Read the model definition and answer for the solid it produces. Units are mm, in the model's axes. Round coordinates to 2 decimals unless told otherwise and drop trailing zeros. Write each loop counter-clockwise with the first axis right and the second up, starting at its lowest first coordinate (ties: lowest second). Pieces come first, ordered by that corner, then holes. Notation, with made-up numbers: (-25.75, 89) - (-21.75, 89) arc R18 cw to (-21.75, 118) - close; hole circle Ø3 at (88, 43.5). An arc over 180 degrees is marked (long way). Answer as CSV lines item,"result". Start each with the question number.
1) Find section B-B on z = 57. Determine the outline of the cut face in (x, y), then the cut area to 3 significant figures.
2) Consider line 1 along Y through (x, z) = (1.8, 78.25); line 2 along Z through (x, y) = (3.55, 5); line 3 along Y through (x, z) = (7, 35.5). Determine where each line is inside the solid, lowest interval first.
3) Each of these flat-tipped pins is pushed along its axis until it touches: pin 1 (1.5 mm diameter, centred on y = 5, z = 8.25, fed in from -X); pin 2 (2 mm diameter, centred on x = 4.25, y = 40.1, fed in from -Z); pin 3 (0.5 mm diameter, centred on y = 34, z = 40.5, fed in from +X). Where does it stop, or does it pass through?
4) Find section A-A on x = 7.25. Determine the outline of the cut face in (y, z).
from build123d import *

# Parameters (mm, degrees)
BOSS_EXTRUDE1_DEPTH            = 86.5
M3X0_5_TAPPED_HOLE2_AT_2_COUNT = 2
M3X0_5_TAPPED_HOLE2_AT_2_PITCH = 23.4
M3X0_5_TAPPED_HOLE1_AT_2_COUNT = 2
M3X0_5_TAPPED_HOLE1_AT_2_PITCH = 46.8


with BuildPart() as part:
    # Sketch1 → Boss-Extrude1 (new body)
    with BuildSketch(Plane.XY):
        Polygon((0, 0), (0, 56.8), (8.5, 56.8), (8.5, 46.8), (2.5, 46.8), (2.5, 45.1), (8.5, 45.1), (8.5, 35.1), (2.5, 35.1), (2.5, 33.4), (8.5, 33.4), (8.5, 23.4), (2.5, 23.4), (2.5, 21.7), (8.5, 21.7), (8.5, 11.7), (2.5, 11.7), (2.5, 10), (8.5, 10), (8.5, 0), align=None)
    extrude(amount=BOSS_EXTRUDE1_DEPTH)

    # Sketch4 → M3x0.5 Tapped Hole2 (revolve, cut)
    with BuildSketch(Plane(origin=(4.25, 40.1, 86.5), x_dir=(0, -1, 0), z_dir=(1, 0, 0))):
        Polygon((0, 0), (0, 5.751075774), (1.25, 5), (1.25, 0), align=None)
    m3x0_5_tapped_hole2 = revolve(axis=Axis((4.25, 40.1, 92.85), (0, 0, -1)), mode=Mode.SUBTRACT)

    # M3x0.5 Tapped Hole2 at 2: M3x0.5 Tapped Hole2 ×2
    with Locations(*[(0, -i * M3X0_5_TAPPED_HOLE2_AT_2_PITCH, 0) for i in range(1, M3X0_5_TAPPED_HOLE2_AT_2_COUNT)]):
        add(m3x0_5_tapped_hole2, mode=Mode.SUBTRACT)

    # Mirror1: M3x0.5 Tapped Hole2 across plane
    add(m3x0_5_tapped_hole2.mirror(Plane.XY.offset(43.25)), mode=Mode.SUBTRACT)

    # Mirror1 copy 1 sketch → Mirror1 copy 1 (revolve, cut)
    with BuildSketch(Plane(origin=(4.25, 16.7, 0), x_dir=(0, -1, 0), z_dir=(1, 0, 0))):
        Polygon((0, 0), (0, -5.751075774), (1.25, -5), (1.25, 0), align=None)
    revolve(axis=Axis((4.25, 16.7, -6.35), (0, 0, -1)), mode=Mode.SUBTRACT)

    # Sketch11 → M3x0.5 Tapped Hole1 (revolve, cut)
    with BuildSketch(Plane(origin=(0, 5, 8.25), x_dir=(0, 0, 1), z_dir=(0, 1, 0))):
        Polygon((0, 0), (0, 5.751075774), (1.25, 5), (1.25, 0), align=None)
    m3x0_5_tapped_hole1 = revolve(axis=Axis((-6.35, 5, 8.25), (1, 0, 0)), mode=Mode.SUBTRACT)

    # M3x0.5 Tapped Hole1 at 2: M3x0.5 Tapped Hole1 ×2
    with Locations(*[(0, i * M3X0_5_TAPPED_HOLE1_AT_2_PITCH, 0) for i in range(1, M3X0_5_TAPPED_HOLE1_AT_2_COUNT)]):
        add(m3x0_5_tapped_hole1, mode=Mode.SUBTRACT)

    # Mirror2: M3x0.5 Tapped Hole1 across plane
    add(m3x0_5_tapped_hole1.mirror(Plane(origin=(0, 0, 43.25), x_dir=(1, 0, 0), z_dir=(0, 0, -1))), mode=Mode.SUBTRACT)

    # Mirror2 copy 1 sketch → Mirror2 copy 1 (revolve, cut)
    with BuildSketch(Plane(origin=(0, 51.8, 78.25), x_dir=(0, 0, -1), z_dir=(0, 1, 0))):
        Polygon((0, 0), (0, -5.751075774), (1.25, -5), (1.25, 0), align=None)
    revolve(axis=Axis((-6.35, 51.8, 78.25), (-1, 0, 0)), mode=Mode.SUBTRACT)


solid = part.part
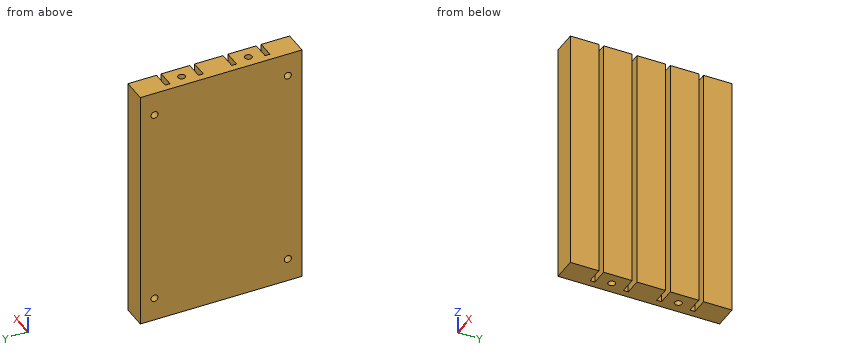
Check values:
1,outline,"(0, 0) - (8.5, 0) - (8.5, 10) - (2.5, 10) - (2.5, 11.7) - (8.5, 11.7) - (8.5, 21.7) - (2.5, 21.7) - (2.5, 23.4) - (8.5, 23.4) - (8.5, 33.4) - (2.5, 33.4) - (2.5, 35.1) - (8.5, 35.1) - (8.5, 45.1) - (2.5, 45.1) - (2.5, 46.8) - (8.5, 46.8) - (8.5, 56.8) - (0, 56.8) - close"
1,area,"442 mm^2"
2,line 1,"y = 0 to 3.75, 6.25 to 50.55, 53.05 to 56.8"
2,line 2,"z = 0 to 7, 9.5 to 77, 79.5 to 86.5"
2,line 3,"y = 0 to 10, 11.7 to 21.7, 23.4 to 33.4, 35.1 to 45.1, 46.8 to 56.8"
3,pin 1,"stops at x = 5.3"
3,pin 2,"stops at z = 5.15"
3,pin 3,"stops at x = 2.5"
4,outline,"(0, 0) - (10, 0) - (10, 86.5) - (0, 86.5) - close; (11.7, 0) - (21.7, 0) - (21.7, 86.5) - (11.7, 86.5) - close; (23.4, 0) - (33.4, 0) - (33.4, 86.5) - (23.4, 86.5) - close; (35.1, 0) - (45.1, 0) - (45.1, 86.5) - (35.1, 86.5) - close; (46.8, 0) - (56.8, 0) - (56.8, 86.5) - (46.8, 86.5) - close"
